from build123d import *

# Parameters (mm, degrees)
SKETCH1_W           = 10
SKETCH1_H           = 6
BOSS_EXTRUDE1_DEPTH = 1
SKETCH2_W           = 1.5
SKETCH2_H           = 2
BOSS_EXTRUDE2_DEPTH = 50


with BuildPart() as part:
    # Sketch1 → Boss-Extrude1 (new body)
    with BuildSketch(Plane(origin=(0, 0, 0), x_dir=(1, 0, 0), z_dir=(0, 1, 0))):
        Rectangle(SKETCH1_W, SKETCH1_H)
    extrude(amount=BOSS_EXTRUDE1_DEPTH)

    # Sketch2 → Boss-Extrude2 (add)
    with BuildSketch(Plane.XZ):
        with Locations((-1.75, 0)):
            Rectangle(SKETCH2_W, SKETCH2_H)
        with Locations((1.75, 0)):
            Rectangle(SKETCH2_W, SKETCH2_H)
    extrude(amount=BOSS_EXTRUDE2_DEPTH)


solid = part.part
Here's how the part is built. I have some questions about the finished solid (model axes, mm). A direction names the side the tool comes from. Coordinates: 2 decimals unless noted, no trailing zeros. Order: outer loops, then holes, each group sorted by start corner. A loop starts at its lowest first (then second) coordinate and runs counter-clockwise, first axis right, second up.
Item 1: If we section it at D-D on x = -3.5: List the corners of the cut face in (y, z) for me, plus the area to 3 significant figures.
Result sheet:
outline: (0, -3) - (1, -3) - (1, 3) - (0, 3) - close
area: 6.00 mm2
Item 2: For faces 1 (the face through (2, -25, 1)), 2 (the face through (2, -25, -1)), 3 (the face through (-2.5, -25, 0)), which set-ups out of +Z, -Z, +X, -X, +Y, -Y let a thin tool reach every point of the face, with its end or its side?
Result sheet:
face 1: +Z, +X, -X, -Y
face 2: -Z, +X, -X, -Y
face 3: +Z, -Z, -X, -Y
Item 3: If we section it at C-C on x = -1.5: List the corners of the cut face in (y, z) for me.
Result sheet:
outline: (-50, -1) - (0, -1) - (0, -3) - (1, -3) - (1, 3) - (0, 3) - (0, 1) - (-50, 1) - close
Item 4: I need wall thicknesses on line 1 (X direction, y = -48, z = 0.75); line 2 (Z direction, x = 1.25, y = -13.5); line 3 (Y direction, x = -4, z = 1.75). Which ranges of each line are inside material? Lowest first, please.
Result sheet:
line 1: x = -2.5 to -1, 1 to 2.5
line 2: z = -1 to 1
line 3: y = 0 to 1
Item 5: If we section it at B-B on y = -4.5: List the corners of the cut face in (x, z) for me, plus the area to 3 significant figures.
Result sheet:
outline: (-2.5, -1) - (-1, -1) - (-1, 1) - (-2.5, 1) - close; (1, -1) - (2.5, -1) - (2.5, 1) - (1, 1) - close
area: 6.00 mm2
Item 6: If we section it at A-A on z = 0.1: List the corners of the cut face in (x, y) for me.
Result sheet:
outline: (-5, 0) - (-2.5, 0) - (-2.5, -50) - (-1, -50) - (-1, 0) - (1, 0) - (1, -50) - (2.5, -50) - (2.5, 0) - (5, 0) - (5, 1) - (-5, 1) - close
Item 7: For P1, Ø1.2, axis at x = -1.5, y = -36, coming from the -Z side; P2, Ø3, axis at x = -2, y = -6.5, coming from the +Z side; P3, Ø1.6, axis at y = -28.5, z = 0, coming from the +X side, each with a flat end and sliding along its axis, tell me the tip position at first contact or that it passes through.
Result sheet:
P1: stops at z = -1
P2: stops at z = 1
P3: stops at x = 2.5
